Check sheet for the modelled part. Datum: model origin and axes. Units: mm. A direction names the side the tool comes from. Round coordinates to 2 decimals unless told otherwise and drop trailing zeros. Write each loop counter-clockwise with the first axis right and the second up, starting at its lowest first coordinate (ties: lowest second). Pieces come first, ordered by that corner, then holes. Notation, with made-up numbers: M 14.5,19.5 L 19.5,19.5 A25 cw 19.5,49.5 Z; hole C 57,11 d3. An arc over 180 degrees is marked long. One line per item, written item: value.
from build123d import *

# Parameters (mm, degrees)
BOSS_EXTRUDE1_START       = 10
SKETCH1_R                 = 1.15
BOSS_EXTRUDE1_DEPTH       = 76
SKETCH2_W                 = 6
SKETCH2_H                 = 16.4
CUT_EXTRUDE1_DEPTH        = 76
BOSS_EXTRUDE2_START       = -47.8
BOSS_EXTRUDE2_DEPTH       = 37.686187853
BOSS_EXTRUDE2_START_2     = -51.8
BOSS_EXTRUDE2_2_OUTLINE_W = 9.85
BOSS_EXTRUDE2_2_OUTLINE_H = 20
BOSS_EXTRUDE2_2_DEPTH     = 12.300000091
BOSS_EXTRUDE2_START_3     = -57.8
BOSS_EXTRUDE2_3_OUTLINE_R = 1.15
BOSS_EXTRUDE2_3_DEPTH     = 3
BOSS_EXTRUDE2_START_4     = 15.2
BOSS_EXTRUDE2_4_OUTLINE_R = 1.15
BOSS_EXTRUDE2_4_DEPTH     = 3
BOSS_EXTRUDE2_START_5     = -27.8
BOSS_EXTRUDE2_5_OUTLINE_W = 6
BOSS_EXTRUDE2_5_OUTLINE_H = 5
BOSS_EXTRUDE2_5_DEPTH     = 16
BOSS_EXTRUDE2_START_6     = -11.8
BOSS_EXTRUDE2_6_DEPTH     = 1.69328026
BOSS_EXTRUDE2_START_7     = -2
BOSS_EXTRUDE2_7_OUTLINE_W = 3
BOSS_EXTRUDE2_7_OUTLINE_H = 10
BOSS_EXTRUDE2_7_DEPTH     = 22
BOSS_EXTRUDE2_8_DEPTH     = 2
BOSS_EXTRUDE2_START_8     = -39.951533137
BOSS_EXTRUDE2_9_OUTLINE_W = 10
BOSS_EXTRUDE2_9_OUTLINE_H = 25.30671974
BOSS_EXTRUDE2_9_DEPTH     = 14.849242405
CHAMFER1_SIZE             = 10
CHAMFER2_SIZE             = 4
CHAMFER3_SIZE             = 4
SKETCH4_W                 = 5
SKETCH4_H                 = 3.2
CUT_EXTRUDE2_DEPTH        = 17
SKETCH5_W                 = 92.220715814
SKETCH5_H                 = 108.753281114
CUT_EXTRUDE3_DEPTH        = 17
BOSS_EXTRUDE3_DEPTH       = 3
BOSS_EXTRUDE4_DEPTH       = 3
CUT_EXTRUDE5_DEPTH        = 26
FILLET1_R                 = 0.5
FILLET2_R                 = 8
CHAMFER4_SIZE             = 6
CHAMFER6_SIZE             = 3.5
BOSS_EXTRUDE6_DEPTH       = 20
CUT_EXTRUDE10_DEPTH       = 34
SKETCH14_W                = 6.88450438
SKETCH14_H                = 12.178080633
CUT_EXTRUDE11_DEPTH       = 5
FILLET3_R                 = 0.5


with BuildPart() as part:
    # Sketch1 → Boss-Extrude1 (new body)
    with BuildSketch(Plane(origin=(0, 0, -57.8), x_dir=(-1, 0, 0), z_dir=(0, 0, -1)).offset(BOSS_EXTRUDE1_START)):
        with BuildLine():
            Line((39, 25), (-18.2, 25))
            Line((-18.2, 25), (-18.2, 20))
            Line((-18.2, 20), (39, 20))
            ThreePointArc((39, 20), (41.5, 22.5), (39, 25))
        make_face()
        with Locations((39, 22.5)):
            Circle(SKETCH1_R, mode=Mode.SUBTRACT)
    extrude(amount=BOSS_EXTRUDE1_DEPTH)

    # Sketch2 → Cut-Extrude1 (cut)
    with BuildSketch(Plane(origin=(0, 25, 0), x_dir=(1, 0, 0), z_dir=(0, 1, 0))):
        with Locations((15.2, 105.8)):
            Rectangle(SKETCH2_W, SKETCH2_H)
    extrude(amount=-CUT_EXTRUDE1_DEPTH, mode=Mode.SUBTRACT)

    # Chamfer1
    chamfer1_edges = [part.edges().sort_by_distance(p)[0] for p in [
        (18.2, 22.5, -143.8),
        (18.2, 22.5, -67.8),
    ]]
    chamfer(chamfer1_edges, length=CHAMFER1_SIZE)

    # Chamfer2
    chamfer2_edges = [part.edges().sort_by_distance(p)[0] for p in [
        (18.2, 25, -87.7),
        (18.2, 25, -123.9),
    ]]
    chamfer(chamfer2_edges, length=CHAMFER2_SIZE)

    # Sketch4 → Cut-Extrude2 (cut)
    with BuildSketch(Plane(origin=(0, 25, 0), x_dir=(1, 0, 0), z_dir=(0, 1, 0))):
        with Locations((-39, 69.4)):
            Rectangle(SKETCH4_W, SKETCH4_H)
        with Locations((-39, 142.2)):
            Rectangle(SKETCH4_W, SKETCH4_H)
    extrude(amount=-CUT_EXTRUDE2_DEPTH, mode=Mode.SUBTRACT)

    # Sketch5 → Cut-Extrude3 (cut)
    with BuildSketch(Plane(origin=(0, 25, 0), x_dir=(1, 0, 0), z_dir=(0, 1, 0))):
        with Locations((-7.000216009, 117.176640557)):
            Rectangle(SKETCH5_W, SKETCH5_H)
    extrude(amount=-CUT_EXTRUDE3_DEPTH, mode=Mode.SUBTRACT)


with BuildPart() as body_2:
    # Boss-Extrude2: read off the stored shape, not the designer's step
    # Boss-Extrude2 outline → Boss-Extrude2 (new body)
    with BuildSketch(Plane.XY.offset(BOSS_EXTRUDE2_START)):
        Polygon((18.2, -2), (18.2, 20), (11.34684114, 20), (11.34684114, 0), (-11.35315886, 0), (-11.35315886, 20), (-15.5, 20), (-20, 15.5), (-20, 0), (-38.5, 0), (-38.5, 20), (-41.5, 20), (-41.5, -2), align=None)
    extrude(amount=BOSS_EXTRUDE2_DEPTH)

    # Boss-Extrude2 2 outline → Boss-Extrude2 2 (add)
    with BuildSketch(Plane.XY.offset(BOSS_EXTRUDE2_START_2)):
        with Locations((6.42184114, 10)):
            Rectangle(BOSS_EXTRUDE2_2_OUTLINE_W, BOSS_EXTRUDE2_2_OUTLINE_H)
        Polygon((-1.50315886, 0), (-1.50315886, 20), (-15.5, 20), (-20, 15.5), (-20, 0), align=None)
    extrude(amount=BOSS_EXTRUDE2_2_DEPTH)

    # Boss-Extrude2 5 outline → Boss-Extrude2 5 (add)
    with BuildSketch(Plane.XY.offset(BOSS_EXTRUDE2_START_5)):
        with Locations((15.2, 22.5)):
            Rectangle(BOSS_EXTRUDE2_5_OUTLINE_W, BOSS_EXTRUDE2_5_OUTLINE_H)
    extrude(amount=BOSS_EXTRUDE2_5_DEPTH)

    # Boss-Extrude2 6 outline → Boss-Extrude2 6 (add)
    with BuildSketch(Plane.XY.offset(BOSS_EXTRUDE2_START_6)):
        Polygon((-11.35315886, 0), (-11.35315886, 20), (-15.5, 20), (-20, 15.5), (-20, 0), align=None)
    extrude(amount=BOSS_EXTRUDE2_6_DEPTH)



with BuildPart() as body_3:
    # Boss-Extrude2 3 outline → Boss-Extrude2 3 (new body)
    with BuildSketch(Plane.XY.offset(BOSS_EXTRUDE2_START_3)):
        with BuildLine():
            Line((1.49684114, 0), (1.49684114, 20))
            Line((1.49684114, 20), (-36.5, 20))
            Line((-36.5, 20), (-36.5, 23))
            ThreePointArc((-36.5, 23), (-37.085786438, 24.414213562), (-38.5, 25))
            Line((-38.5, 25), (-39.5, 25))
            ThreePointArc((-39.5, 25), (-40.914213562, 24.414213562), (-41.5, 23))
            Line((-41.5, 23), (-41.5, 20))
            Line((-41.5, 20), (-38.5, 20))
            Line((-38.5, 20), (-38.5, 0))
            Line((-38.5, 0), (1.49684114, 0))
        make_face()
        with Locations((-39, 22.5)):
            Circle(BOSS_EXTRUDE2_3_OUTLINE_R, mode=Mode.SUBTRACT)
    extrude(amount=BOSS_EXTRUDE2_3_DEPTH)


with BuildPart() as body_4:
    # Boss-Extrude2 4 outline → Boss-Extrude2 4 (new body)
    with BuildSketch(Plane.XY.offset(BOSS_EXTRUDE2_START_4)):
        with BuildLine():
            Line((1.49684114, 0), (1.49684114, 20))
            Line((1.49684114, 20), (-36.5, 20))
            Line((-36.5, 20), (-36.5, 23))
            ThreePointArc((-36.5, 23), (-37.085786438, 24.414213562), (-38.5, 25))
            Line((-38.5, 25), (-39.5, 25))
            ThreePointArc((-39.5, 25), (-40.914213562, 24.414213562), (-41.5, 23))
            Line((-41.5, 23), (-41.5, 20))
            Line((-41.5, 20), (-38.5, 20))
            Line((-38.5, 20), (-38.5, 0))
            Line((-38.5, 0), (1.49684114, 0))
        make_face()
        with Locations((-39, 22.5)):
            Circle(BOSS_EXTRUDE2_4_OUTLINE_R, mode=Mode.SUBTRACT)
    extrude(amount=BOSS_EXTRUDE2_4_DEPTH)


with BuildPart() as body_2_1:
    add(body_2.part)

    add(body_3.part)  # Boss-Extrude2 7 merges body 3

    add(body_4.part)  # Boss-Extrude2 7 merges body 4
    # Boss-Extrude2 7 outline → Boss-Extrude2 7 (add)
    with BuildSketch(Plane(origin=(0, 0, 0), x_dir=(1, 0, 0), z_dir=(0, 1, 0)).offset(BOSS_EXTRUDE2_START_7)):
        Polygon((18.2, 47.8), (8.2, 57.8), (1.49684114, 57.8), (1.49684114, 47.8), align=None)
        with BuildLine():
            Line((18.2, -8.2), (18.2, 10.113812147))
            Line((18.2, 10.113812147), (11.34684114, 10.113812147))
            ThreePointArc((11.34684114, 10.113812147), (0.0047491, -15.199999258), (-11.35315886, 10.10671974))
            Line((-11.35315886, 10.10671974), (-20, 10.10671974))
            Line((-20, 10.10671974), (-20, -15.2))
            Line((-20, -15.2), (-38.5, -15.2))
            Line((-38.5, -15.2), (-38.5, 10.113812147))
            Line((-38.5, 10.113812147), (-41.5, 10.113812147))
            Line((-41.5, 10.113812147), (-41.5, -18.2))
            Line((-41.5, -18.2), (8.2, -18.2))
            Line((8.2, -18.2), (18.2, -8.2))
        make_face()
        with Locations((-40, 52.8)):
            Rectangle(BOSS_EXTRUDE2_7_OUTLINE_W, BOSS_EXTRUDE2_7_OUTLINE_H)
    extrude(amount=BOSS_EXTRUDE2_7_DEPTH)

    # Boss-Extrude2 8 outline → Boss-Extrude2 8 (add)
    with BuildSketch(Plane(origin=(0, 0, 0), x_dir=(1, 0, 0), z_dir=(0, 1, 0)).offset(BOSS_EXTRUDE2_START_7)):
        Polygon((1.49684114, 47.8), (1.49684114, 57.8), (-38.5, 57.8), (-38.5, 47.8), (-20, 47.8), align=None)
        with BuildLine():
            Line((11.34684114, 10.113812147), (-38.5, 10.113812147))
            Line((-38.5, 10.113812147), (-38.5, -15.2))
            Line((-38.5, -15.2), (-20, -15.2))
            Line((-20, -15.2), (-20, 10.10671974))
            Line((-20, 10.10671974), (-11.35315886, 10.10671974))
            ThreePointArc((-11.35315886, 10.10671974), (0.0047491, -15.199999258), (11.34684114, 10.113812147))
        make_face()
    extrude(amount=BOSS_EXTRUDE2_8_DEPTH)

    # Boss-Extrude2 9 outline → Boss-Extrude2 9 (cut)
    with BuildSketch(Plane(origin=(0, 0, 0), x_dir=(0.7071067811865474, 0.7071067811865477, 0), z_dir=(0.7071067811865476, -0.7071067811865476, 0)).offset(BOSS_EXTRUDE2_START_8)):
        with Locations((0, 2.54664013)):
            Rectangle(BOSS_EXTRUDE2_9_OUTLINE_W, BOSS_EXTRUDE2_9_OUTLINE_H)
    extrude(amount=BOSS_EXTRUDE2_9_DEPTH, mode=Mode.SUBTRACT)

    # Chamfer3
    chamfer3_edges = [body_2_1.edges().sort_by_distance(p)[0] for p in [
        (18.2, 25, -19.8),
    ]]
    chamfer(chamfer3_edges, length=CHAMFER3_SIZE)

    # Sketch6 → Boss-Extrude3 (add)
    with BuildSketch(Plane.XY.offset(18.2)):
        Polygon((-36.5, 23), (-33.5, 20), (-37.431383681, 19.25446979), align=None)
    extrude(amount=-BOSS_EXTRUDE3_DEPTH)

    # Sketch7 → Boss-Extrude4 (add)
    with BuildSketch(Plane(origin=(0, 0, -57.8), x_dir=(-1, 0, 0), z_dir=(0, 0, -1))):
        Polygon((36.5, 23), (33.5, 20), (37.220279648, 19.344567212), align=None)
    extrude(amount=-BOSS_EXTRUDE4_DEPTH)

    # Sketch8 → Cut-Extrude5 (cut)
    with BuildSketch(Plane(origin=(0, 20, 0), x_dir=(1, 0, 0), z_dir=(0, 1, 0))):
        Polygon((18.2, 11.8), (14.7, 8.3), (14.7, -21.501109559), (24.075722879, -13.334137275), (24.580871836, 10.828821177), align=None)
    extrude(amount=-CUT_EXTRUDE5_DEPTH, mode=Mode.SUBTRACT)

    # Fillet1
    fillet1_edges = [body_2_1.edges().sort_by_distance(p)[0] for p in [
        (14.7, 10, -3.866522986),
        (14.7, 10, 3.866522986),
    ]]
    fillet(fillet1_edges, radius=FILLET1_R)

    # Fillet2
    fillet2_edges = [body_2_1.edges().sort_by_distance(p)[0] for p in [
        (-38.5, 0, -19.8),
    ]]
    fillet(fillet2_edges, radius=FILLET2_R)

    # Chamfer4
    chamfer4_edges = [body_2_1.edges().sort_by_distance(p)[0] for p in [
        (-41.5, -2, -19.8),
    ]]
    chamfer(chamfer4_edges, length=CHAMFER4_SIZE)

    # Chamfer6
    chamfer6_edges = [body_2_1.edges().sort_by_distance(p)[0] for p in [
        (13.2, -2, -52.8),
        (11.45, -2, 14.95),
    ]]
    chamfer(chamfer6_edges, length=CHAMFER6_SIZE)

    # Sketch12 → Boss-Extrude6 (add)
    with BuildSketch(Plane(origin=(0, 0, 0), x_dir=(1, 0, 0), z_dir=(0, 1, 0))):
        with BuildLine():
            Line((0, -16.836473334), (-10.35781432, -16.574633061))
            Line((-10.35781432, -16.574633061), (-15.5, -4.91441497))
            Line((-15.5, -4.91441497), (-15.5, 9.8))
            Line((-15.5, 9.8), (-11.35315886, 10.10671974))
            Line((-11.35315886, 10.10671974), (-11.35315886, 2.5302757))
            ThreePointArc((-11.35315886, 2.5302757), (0.007539589, -15.199997726), (11.34684114, 2.543967596))
            Line((11.34684114, 2.543967596), (11.34684114, 10.113812147))
            Line((11.34684114, 10.113812147), (14.7, 8.3))
            Line((14.7, 8.3), (14.7, -11.7))
            Line((14.7, -11.7), (4.492447971, -17.057179979))
            Line((4.492447971, -17.057179979), (0, -16.836473334))
        make_face()
    extrude(amount=BOSS_EXTRUDE6_DEPTH)

    # Sketch13 → Cut-Extrude10 (cut)
    with BuildSketch(Plane(origin=(0, 20, 0), x_dir=(1, 0, 0), z_dir=(0, 1, 0))):
        Polygon((14.7, 8.3), (12.2, 5.521362845), (12.2, -21.090159973), (18.418004591, -14.179128538), align=None)
    extrude(amount=-CUT_EXTRUDE10_DEPTH, mode=Mode.SUBTRACT)

    # Sketch14 → Cut-Extrude11 (cut)
    with BuildSketch(Plane(origin=(6.069669914, -8.583809512, 6.069669914), x_dir=(0.8660254037844393, 0.40824829046386313, -0.28867513459481114), z_dir=(0.49999999999999906, -0.7071067811865493, 0.49999999999999833))):
        with Locations((7.600391897, 9.638669458)):
            Rectangle(SKETCH14_W, SKETCH14_H)
    extrude(amount=CUT_EXTRUDE11_DEPTH, mode=Mode.SUBTRACT)

    # Fillet3
    # the kernel refuses this fillet: 0.5 mm, written as the material it takes off along each edge
    with BuildSketch(Plane(origin=(12.2, 27.361092772, 5.422131518), x_dir=(0, 0, 1), z_dir=(0, -1, 0))) as fillet3_piece_1:
        with BuildLine():
            CenterArc((2.944437109, 0.5), FILLET3_R, 115.841932763, 154.158067237)
            ThreePointArc((2.726492162, 0.95), (1.39076711, 0.396014873), (0, 0))
            Line((0, 0), (2.944437109, 0))
        make_face()
    extrude(amount=27.361092772, mode=Mode.SUBTRACT)
    with BuildSketch(Plane(origin=(12.2, 27.189458898, -0.022131518), x_dir=(0, 0, -1), z_dir=(0, -1, 0))) as fillet3_piece_2:
        with BuildLine():
            CenterArc((2.875783559, -0.5), FILLET3_R, 90, 134.936099196)
            ThreePointArc((2.521836078, -0.85315886), (1.28369596, -0.359250606), (0, 0))
            Line((0, 0), (2.875783559, 0))
        make_face()
    extrude(amount=27.189458898, mode=Mode.SUBTRACT)


solid = body_2_1.part
Q1. Depth check by flat-ended pin: P1, Ø12, axis at x = 10, y = 8, coming from the -Z side; P2, Ø6, axis at y = 13, z = 1, coming from the +X side; P3, Ø10, axis at x = -27.5, z = 2, coming from the +Y side; P4, Ø2, axis at x = 1.5, z = -35.5, coming from the +Y side. Enter the tip coordinate at first touch or a pass-through.
Completed:
P1: z = -57.8
P2: x = -11.58
P3: y = 0.25
P4: y = 0
Q2. Sectioned sample at D-D on z = -42. Enter the section's corners in (x, y).
Completed:
outline: M -41.5,4 L -35.5,-2 L 18.2,-2 L 18.2,20 L 1.5,20 L 1.5,0 L -1.5,0 L -1.5,20 L -15.5,20 L -20,15.5 L -20,0 L -30.5,0 A8 cw -38.5,8 L -38.5,20 L -41.5,20 Z
Q3. Draft check along X on faces 1 (the flat face through (-35, 21.5, -56.3)), 2 (the cylindrical face through (-40.9, 24.43, 16.68)), 3 (the cylindrical face through (-5.59, 9.86, 13.88)). Enter one of: pulls with the +X half, pulls with the -X half, needs draft (parallel to the pull), parting line crosses it, or undercut.
Completed:
face 1: pulls with the +X half
face 2: pulls with the -X half
face 3: undercut
Q4. Sectioned sample at C-C on y = 9.75. Enter the section's corners in (x, z), and give its area (3 significant figures).
Completed:
outline: M -41.5,-57.8 L 8.2,-57.8 L 18.2,-47.8 L 18.2,-11.8 L 14.7,-8.3 L 12.2,-5.52 L 12.2,-2.9 A0.5 ccw 11.35,-2.54 L 11.35,-39.5 L 1.5,-39.5 L 1.5,-54.8 L -38.5,-54.8 L -38.5,15.2 L -20,15.2 L -20,-51.8 L -1.5,-51.8 L -1.5,-39.5 L -11.35,-39.5 L -11.35,-2.53 A12.5 cw 11.25,8.15 A0.5 ccw 12.2,8.37 L 12.2,14.2 L 8.2,18.2 L -41.5,18.2 Z
area: 1,710 mm^2
Q5. Scan lines: line 1 (Y direction, x = -39, z = -56.9); line 2 (Z direction, x = -26, y = 1); line 3 (X direction, y = 8, z = -50). Record each from-to range of solid material in increasing order. Write a range as [from, to].
Completed:
line 1: [1.5, 21.35], [23.65, 25]
line 2: [-57.8, -54.8], [15.2, 18.2]
line 3: [-41.5, -38.5], [-20, -1.5], [1.5, 16]
Q6. Sectioned sample at A-A on z = 2.7. Enter the section's corners in (x, y), and give its area (3 significant figures).
Completed:
outline: M -41.5,4 L -35.5,-2 L 12.2,-2 L 12.2,0 L -12.5,0 L -12.5,20 L -15.5,20 L -20,15.5 L -20,0 L -30.5,0 A8 cw -38.5,8 L -38.5,20 L -41.5,20 Z
area: 303 mm^2
Q7. Sectioned sample at B-B on x = -16.5. Enter the section's corners in (y, z), and give its area (4 significant figures).
Completed:
outline: M -2,-57.8 L 20,-57.8 L 20,-54.8 L 0,-54.8 L 0,-51.8 L 19,-51.8 L 19,15.2 L 20,15.2 L 20,18.2 L -2,18.2 Z
area: 1,545 mm^2
Q8. Access from +Z, -Z, +X, -X, +Y, -Y to the whole of each face (thin tool, end or side, straight path). Record for faces 4 (the flat face through (-17.8, 17.7, -17.8)), 5 (the flat face through (18.2, 9, -30)), 6 (the flat face through (-40, 20, -20)).
Completed:
face 4: +Y
face 5: +Z, -Z, +X, +Y, -Y
face 6: -X, +Y
